Model file for the job. Use its own axes, mm. A direction names the side the tool comes from. Give positions to 0.01 mm unless a question says otherwise; leave off trailing zeros. Order: outer loops, then holes, each group sorted by start corner. A loop starts at its lowest first (then second) coordinate and runs counter-clockwise, first axis right, second up. Notation, with made-up numbers: (75.5, 36.25) -> (93.5, 36.25) arc R25 cw to (93.5, 50.25) -> close; hole circle Ø4 at (14, 9). An arc over 180 degrees is marked (long way). Answer in a Markdown table with one row per item. Add a question column.
from build123d import *

# Parameters (mm, degrees)
SKETCH1_R           = 21
BOSS_EXTRUDE1_DEPTH = 34
SKETCH2_R           = 7.5
BOSS_EXTRUDE2_DEPTH = 1.25
SKETCH3_R           = 2.955
BOSS_EXTRUDE3_DEPTH = 14.85
CUT_EXTRUDE1_START  = -11
CUT_EXTRUDE1_DEPTH  = 11
SKETCH5_R           = 0.625
CUT_EXTRUDE2_DEPTH  = 20
SKETCH6_R           = 1.25
CUT_EXTRUDE3_DEPTH  = 4
CIRPATTERN1_COUNT   = 3
BOSS_EXTRUDE4_START = -29.27
BOSS_EXTRUDE4_DEPTH = 12.68
SKETCH10_R          = 4
CUT_EXTRUDE4_DEPTH  = 1.66


with BuildPart() as part:
    # Sketch1 → Boss-Extrude1 (new body)
    with BuildSketch(Plane.XY):
        Circle(SKETCH1_R)
    extrude(amount=BOSS_EXTRUDE1_DEPTH)

    # Sketch2 → Boss-Extrude2 (add)
    with BuildSketch(Plane.XY.offset(34)):
        Circle(SKETCH2_R)
    extrude(amount=BOSS_EXTRUDE2_DEPTH)

    # Sketch3 → Boss-Extrude3 (add)
    with BuildSketch(Plane.XY.offset(35.25)):
        Circle(SKETCH3_R)
    extrude(amount=BOSS_EXTRUDE3_DEPTH)

    # Sketch4 → Cut-Extrude1 (cut)
    with BuildSketch(Plane.XY.offset(50.1).offset(CUT_EXTRUDE1_START)):
        with BuildLine():
            Line((-2.518928344, 1.545), (2.518928344, 1.545))
            ThreePointArc((2.518928344, 1.545), (0, 2.955), (-2.518928344, 1.545))
        make_face()
    extrude(amount=CUT_EXTRUDE1_DEPTH, mode=Mode.SUBTRACT)

    # Sketch5 → Cut-Extrude2 (cut)
    with BuildSketch(Plane.XY.offset(50.1)):
        Circle(SKETCH5_R)
    extrude(amount=-CUT_EXTRUDE2_DEPTH, mode=Mode.SUBTRACT)

    # Sketch6 → Cut-Extrude3 (cut)
    with BuildSketch(Plane.XY.offset(34)):
        with Locations((0, -15)):
            Circle(SKETCH6_R)
    cut_extrude3 = extrude(amount=-CUT_EXTRUDE3_DEPTH, mode=Mode.SUBTRACT)

    # CirPattern1: Cut-Extrude3 ×3 about axis
    cirpattern1_axis = Axis((0, 0, 0), (0, 0, 1))
    for i in range(1, CIRPATTERN1_COUNT):
        add(cut_extrude3.rotate(cirpattern1_axis, i * 360 / CIRPATTERN1_COUNT), mode=Mode.SUBTRACT)

    # Sketch9 → Boss-Extrude4 (add)
    with BuildSketch(Plane.XY.offset(34).offset(BOSS_EXTRUDE4_START)):
        with BuildLine():
            Line((-14, 15.652475842), (-14, 29.66))
            Line((-14, 29.66), (14, 29.66))
            Line((14, 29.66), (14, 15.652475842))
            ThreePointArc((14, 15.652475842), (0, 21), (-14, 15.652475842))
        make_face()
    extrude(amount=BOSS_EXTRUDE4_DEPTH)

    # Sketch10 → Cut-Extrude4 (cut)
    with BuildSketch(Plane(origin=(0, 0, 0), x_dir=(-1, 0, 0), z_dir=(0, 0, -1))):
        Circle(SKETCH10_R)
    extrude(amount=-CUT_EXTRUDE4_DEPTH, mode=Mode.SUBTRACT)


solid = part.part
Item 1: Wall check: line 1 (Y direction, x = 0, z = 32.4) (3 decimals); line 2 (Z direction, x = -4.5, y = 3); line 3 (Z direction, x = 0, y = 21.5). Give the ranges that are in metal, low to high.
Item 2: Pin check, flat tips, straight feed: pin 1 Ø8 at (y, z) = (11, 8) entering from -X; pin 2 Ø1.6 at (x, y) = (1, 2.5) entering from +Z; pin 3 Ø6 at (y, z) = (17, 6.5) entering from +X; pin 4 Ø6.5 at (x, y) = (0, 0) entering from +Z. Stop position of each tip, or through.
Item 3: Saw through at B-B on z = 6. List the corners of the cut face in (x, y).
Item 4: Saw through at A-A on y = -6.5. List the corners of the cut face in (x, z), plus the area to 3 significant figures.
Item 5: Two-plate mould, pull along Y, no slides. Class faces 5 (the flat face through (0, 1.545, 45)), 6 (the cylindrical face through (-13.912, 8.345, 32.028)), 7 (the cylindrical face through (-7.493, 0.33, 34.616)): pulls with the +Y half, pulls with the -Y half, needs draft (parallel to the pull), parting line crosses it, or undercut.
Item 6: Saw through at C-C on x = 10. List the corners of the cut face in (y, z).
Item 7: Saw through at D-D on y = 22. List the corners of the cut face in (x, z), plus the area to 3 significant figures.
Item 8: Which spindle directions (+Z, -Z, +X, -X, +Y, -Y) get a long thin tool onto all of the face, cutting with end or side? Do faces 1 (the flat face through (-14, 23, 11)), 2 (the flat face through (0, 0, 30.1)), 3 (the cylindrical face through (0.867, -3.905, 0.818)), 4 (the flat face through (14, 23, 11)). Say none if no direction does.
Evaluation:
| question | item | result |
|---|---|---|
| 1 | line 1 | y = -21 to -16.25, -13.75 to -0.625, 0.625 to 21 |
| 1 | line 2 | z = 0 to 35.25 |
| 1 | line 3 | z = 4.73 to 17.41 |
| 2 | pin 1 | stops at x = -19.8 |
| 2 | pin 2 | stops at z = 39.1 |
| 2 | pin 3 | stops at x = 15.65 |
| 2 | pin 4 | stops at z = 50.1 |
| 3 | outline | (-14, 15.65) arc R21 ccw (long way) to (14, 15.65) -> (14, 29.66) -> (-14, 29.66) -> close |
| 4 | outline | (-19.97, 0) -> (19.97, 0) -> (19.97, 34) -> (3.74, 34) -> (3.74, 35.25) -> (-3.74, 35.25) -> (-3.74, 34) -> (-19.97, 34) -> close |
| 4 | area | 1,370 mm2 |
| 5 | face 5 | pulls with the +Y half |
| 5 | face 6 | undercut |
| 5 | face 7 | parting line crosses it |
| 6 | outline | (-18.47, 0) -> (18.47, 0) -> (18.47, 4.73) -> (29.66, 4.73) -> (29.66, 17.41) -> (18.47, 17.41) -> (18.47, 34) -> (-18.47, 34) -> close |
| 7 | outline | (-14, 4.73) -> (14, 4.73) -> (14, 17.41) -> (-14, 17.41) -> close |
| 7 | area | 355 mm2 |
| 8 | face 1 | +Z, -Z, -X, +Y |
| 8 | face 2 | +Z |
| 8 | face 3 | -Z |
| 8 | face 4 | +Z, -Z, +X, +Y |
